The listing builds one solid part. Answer for the finished solid, in the listing's coordinates (mm). A direction names the side the tool comes from. Give positions to 0.01 mm unless a question says otherwise; leave off trailing zeros. Order: outer loops, then holes, each group sorted by start corner. A loop starts at its lowest first (then second) coordinate and runs counter-clockwise, first axis right, second up.
```python
from build123d import *

# Parameters (mm, degrees)
F0_R          = 5
F0_R_2        = 0.5
F1_DEPTH      = 10
F2_R          = 3
F3_DEPTH      = 40
F4_R          = 1.75
F5_DEPTH      = 9.001
F5_DEPTH_BACK = 9.001
F6_R          = 10
F7_SIZE2      = 3
F7_SIZE       = 2
F7_2_SIZE2    = 3
F7_2_SIZE     = 2


# Not quite as in the source:
# - a pattern or mirror of a feature is missing from the dataset's text; its kind, count and spacing are read off the source's solid


with BuildPart() as f1:
    # F0 (on Front) → F1 (new body)
    with BuildSketch(Plane.XZ):
        with BuildLine():
            Line((71, 5), (7.4833147735, 5))
            ThreePointArc((7.4833147735, 5), (0, 9), (-7.4833147735, 5))
            Line((-7.4833147735, 5), (-72, 5))
            Line((-72, 5), (-72, -5))
            Line((-72, -5), (-7.4833147735, -5))
            ThreePointArc((-7.4833147735, -5), (0, -9), (7.4833147735, -5))
            Line((7.4833147735, -5), (71, -5))
            Line((71, -5), (71, 5))
        make_face()
        Circle(F0_R, mode=Mode.SUBTRACT)
        with Locations((8, 0)):
            Circle(F0_R_2, mode=Mode.SUBTRACT)
    extrude(amount=F1_DEPTH)

    # F2 (on face) → F3 (cut)
    with BuildSketch(Plane(origin=(-72, 0, 0), x_dir=(0, -1, 0), z_dir=(-1, 0, 0))):
        with Locations((5, 0)):
            Circle(F2_R)
    f3 = extrude(amount=-F3_DEPTH, mode=Mode.SUBTRACT)

    # F3_copies: F3 across plane
    add(f3.mirror(Plane(origin=(0, 0, 0), x_dir=(0, 0, 1), z_dir=(1, 0, 0))), mode=Mode.SUBTRACT)

    # F4 (on Top) → F5 (cut, two sides)
    with BuildSketch(Plane.XY) as f5_sk:
        with Locations((0, -5)):
            Circle(F4_R)
    extrude(amount=-F5_DEPTH, mode=Mode.SUBTRACT)
    extrude(f5_sk.sketch, amount=F5_DEPTH_BACK, mode=Mode.SUBTRACT)

    # F6
    f6_edges = [f1.edges().sort_by_distance(p)[0] for p in [
        (-7.483315, -5, 5),
        (7.483315, -5, 5),
        (7.483315, -5, -5),
        (-7.483315, -5, -5),
    ]]
    fillet(f6_edges, radius=F6_R)

    # F7
    f7_edges = [f1.edges().sort_by_distance(p)[0] for p in [
        (-41.830952, -10, 5),
        (-41.830952, -10, -5),
    ]]
    f7_side = f1.faces().sort_by_distance((41.330952, -10, -3.558716))[0]
    chamfer(f7_edges, length=F7_SIZE, length2=F7_SIZE2, reference=f7_side)

    # F7#2
    f7_2_edges = [f1.edges().sort_by_distance(p)[0] for p in [
        (-41.830952, 0, 5),
        (-41.830952, 0, -5),
    ]]
    f7_2_side = f1.faces().sort_by_distance((41.330952, 0, -3.558716))[0]
    chamfer(f7_2_edges, length=F7_2_SIZE, length2=F7_2_SIZE2, reference=f7_2_side)


solid = f1.part
```
1) For a pull along X with two mould halves and no side action, classify faces 1 (the flat face through (40.9, -1.5, -4)), 2 (the cylindrical face through (-1.75, -4.92, -6.81)), 3 (the cylindrical face through (-1.4, -3.64, -8.89)) as +X half, -X half, draft (parallel to the pull), parting line (faces both ways), or undercut.
Geometry says:
face 1: draft
face 2: undercut
face 3: parting line
2) A tool of negligible diameter and unlimited length cuts with its end or side. For faces 4 (the flat face through (-42, -5, -5)), 5 (the flat face through (40.9, -8.5, -4)), 6 (the flat face through (-41, -5, 5)), from which of +Z, -Z, +X, -X, +Y, -Y can it reach the whole face along a straight path? Write none if from no direction.
Geometry says:
face 4: -Z, -X, +Y, -Y
face 5: -Z, +X, -Y
face 6: +Z, -X, +Y, -Y
3) Find section A-A (x = -44.5). Write down the section's boundary in (y, z), then the cut area to 3 significant figures.
Geometry says:
outline: (-10, -3) - (-7, -5) - (-3, -5) - (0, -3) - (0, 3) - (-3, 5) - (-7, 5) - (-10, 3) - close; hole circle Ø6 at (-5, 0)
area: 59.7 mm2
4) Find section B-B (x = 0). Write down the section's boundary in (y, z).
Geometry says:
outline: (-10, -7) - (-7, -9) - (-6.75, -9) - (-6.75, -5) - (-10, -5) - close; (-10, 5) - (-6.75, 5) - (-6.75, 9) - (-7, 9) - (-10, 7) - close; (-3.25, -9) - (-3, -9) - (0, -7) - (0, -5) - (-3.25, -5) - close; (-3.25, 5) - (0, 5) - (0, 7) - (-3, 9) - (-3.25, 9) - close
5) Given P1, Ø1.2, axis at x = -31, y = -4.5, coming from the -Z side; P2, Ø4.5, axis at x = -37.5, y = -4.5, coming from the +Z side; P3, Ø1.5, axis at y = -3, z = 7, coming from the -X side, each flat-ended and moving along its own axis, determine where each tip first touches the part or whether it passes through.
Geometry says:
P1: stops at z = -5
P2: stops at z = 5
P3: stops at x = -6.82
6) Find section C-C (y = -5). Count the separate pieces of the cut face and the enclosed holes in it, then the cut area to 3 significant figures.
Geometry says:
separate pieces: 2
enclosed holes: 1
area: 940 mm2
7) Find section D-D (x = 23). Write down the section's boundary in (y, z), then the cut area to 3 significant figures.
Geometry says:
outline: (-10, -3) - (-7, -5) - (-3, -5) - (0, -3) - (0, 3) - (-3, 5) - (-7, 5) - (-10, 3) - close
area: 88.0 mm2
8) Straight lines are drawn through the part: probe 1 along Y at (x, z) = (43, 0); probe 2 along Y at (x, z) = (0, 5.75); probe 3 along Z at (x, y) = (-49, -5). For each, find the intervals that lie inside material, in ascending order.
Geometry says:
probe 1: y = -10 to -8, -2 to 0
probe 2: y = -10 to -6.75, -3.25 to 0
probe 3: z = -5 to -3, 3 to 5
